Build history of the part. All positions in model axes, mm. Give positions to 0.01 mm unless a question says otherwise; leave off trailing zeros. Answer as a JSON object with one key per item and string values. Group by question number.
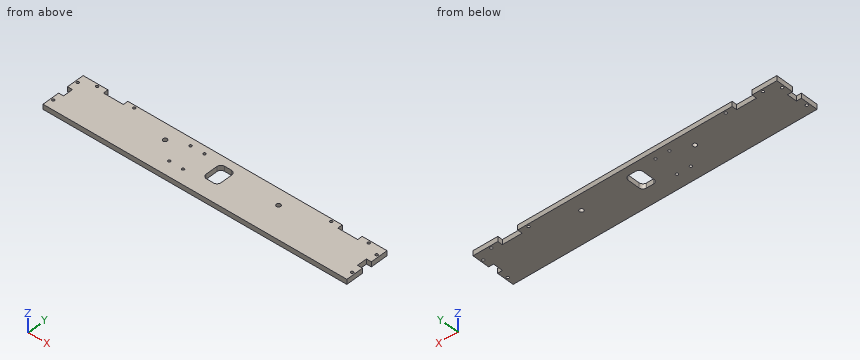
from build123d import *

# Parameters (mm, degrees)
SKETCH1_R           = 1.65
SKETCH1_R_2         = 2.7
BOSS_EXTRUDE1_DEPTH = 6.35
CUT_EXTRUDE1_REACH  = 8.35
SKETCH2_R           = 1.65


with BuildPart() as part:
    # Sketch1 → Boss-Extrude1 (new body)
    with BuildSketch(Plane(origin=(0, 0, 215.9), x_dir=(-1, 0, 0), z_dir=(0, 0, -1))):
        Polygon((50.8, 57.15), (50.8, 50.8), (25.4, 50.8), (25.4, 57.15), (-6.35, 57.15), (-6.35, 34.925), (0, 34.925), (0, 22.225), (-6.35, 22.225), (-6.35, 0), (382.27, 0), (382.27, 22.225), (375.92, 22.225), (375.92, 34.925), (382.27, 34.925), (382.27, 57.15), (350.52, 57.15), (350.52, 50.8), (325.12, 50.8), (325.12, 57.15), align=None)
        with Locations((379.095, 11.1125)):
            Circle(SKETCH1_R, mode=Mode.SUBTRACT)
        with Locations((-3.175, 11.1125)):
            Circle(SKETCH1_R, mode=Mode.SUBTRACT)
        with Locations((379.095, 46.037500912)):
            Circle(SKETCH1_R, mode=Mode.SUBTRACT)
        with Locations((-3.175, 46.037500912)):
            Circle(SKETCH1_R, mode=Mode.SUBTRACT)
        with Locations((314.0075, 53.975)):
            Circle(SKETCH1_R, mode=Mode.SUBTRACT)
        with Locations((61.9125, 53.975)):
            Circle(SKETCH1_R, mode=Mode.SUBTRACT)
        with Locations((361.6325, 53.975)):
            Circle(SKETCH1_R, mode=Mode.SUBTRACT)
        with Locations((14.2875, 53.975)):
            Circle(SKETCH1_R, mode=Mode.SUBTRACT)
        with Locations((260.51, 38.26)):
            Circle(SKETCH1_R_2, mode=Mode.SUBTRACT)
        with Locations((115.41, 38.26)):
            Circle(SKETCH1_R_2, mode=Mode.SUBTRACT)
        with BuildLine():
            Line((192.405, 21.59), (183.515, 21.59))
            ThreePointArc((183.515, 21.59), (179.922897552, 23.077897552), (178.435, 26.67))
            Line((178.435, 26.67), (178.435, 41.91))
            ThreePointArc((178.435, 41.91), (179.922897552, 45.502102448), (183.515, 46.99))
            Line((183.515, 46.99), (192.405, 46.99))
            ThreePointArc((192.405, 46.99), (195.997102448, 45.502102448), (197.485, 41.91))
            Line((197.485, 41.91), (197.485, 26.67))
            ThreePointArc((197.485, 26.67), (195.997102448, 23.077897552), (192.405, 21.59))
        make_face(mode=Mode.SUBTRACT)
    extrude(amount=-BOSS_EXTRUDE1_DEPTH)

    # Sketch2 → Cut-Extrude1 (cut, up to next)
    with BuildSketch(Plane.XY.offset(222.25), mode=Mode.PRIVATE) as cut_extrude1_sk1:
        with Locations((-218.821, 47.9552)):
            Circle(SKETCH2_R)
    cut_extrude1_tool1 = extrude(cut_extrude1_sk1.sketch, amount=-CUT_EXTRUDE1_REACH, mode=Mode.PRIVATE) & part.part
    add(cut_extrude1_tool1.solids().sort_by_distance((-218.821, 47.9552, 222.25))[0], mode=Mode.SUBTRACT)
    # Sketch2 → Cut-Extrude1 (cut, up to next)
    with BuildSketch(Plane.XY.offset(222.25), mode=Mode.PRIVATE) as cut_extrude1_sk2:
        with Locations((-236.601, 47.9552)):
            Circle(SKETCH2_R)
    cut_extrude1_tool2 = extrude(cut_extrude1_sk2.sketch, amount=-CUT_EXTRUDE1_REACH, mode=Mode.PRIVATE) & part.part
    add(cut_extrude1_tool2.solids().sort_by_distance((-236.601, 47.9552, 222.25))[0], mode=Mode.SUBTRACT)
    # Sketch2 → Cut-Extrude1 (cut, up to next)
    with BuildSketch(Plane.XY.offset(222.25), mode=Mode.PRIVATE) as cut_extrude1_sk3:
        with Locations((-236.601, 17.4752)):
            Circle(SKETCH2_R)
    cut_extrude1_tool3 = extrude(cut_extrude1_sk3.sketch, amount=-CUT_EXTRUDE1_REACH, mode=Mode.PRIVATE) & part.part
    add(cut_extrude1_tool3.solids().sort_by_distance((-236.601, 17.4752, 222.25))[0], mode=Mode.SUBTRACT)
    # Sketch2 → Cut-Extrude1 (cut, up to next)
    with BuildSketch(Plane.XY.offset(222.25), mode=Mode.PRIVATE) as cut_extrude1_sk4:
        with Locations((-218.821, 17.4752)):
            Circle(SKETCH2_R)
    cut_extrude1_tool4 = extrude(cut_extrude1_sk4.sketch, amount=-CUT_EXTRUDE1_REACH, mode=Mode.PRIVATE) & part.part
    add(cut_extrude1_tool4.solids().sort_by_distance((-218.821, 17.4752, 222.25))[0], mode=Mode.SUBTRACT)


solid = part.part
(1) Saw through at A-A on z = 220.5. Give the number of separate pieces and of enclosed holes in the cut face, plus the area to 3 significant figures.
(2) Pin check, flat tips, straight feed: pin 1 (2.5 mm diameter, centred on x = -236.6, y = 17.48, fed in from -Z); pin 2 (3 mm diameter, centred on x = -187.5, z = 218, fed in from -Y); pin 3 (2 mm diameter, centred on x = -336.5, z = 221, fed in from +Y); pin 4 (1.9 mm diameter, centred on y = 29, z = 218, fed in from -X). Stop position of each tip, or through.
(3) Probe line 1 along X through (y, z) = (38, 217) (3 decimals); line 2 along X through (y, z) = (52, 219.25); line 3 along X through (y, z) = (42, 216.5). List the from-to ranges inside material, lowest first. Write a range as [from, to].
Calculated:
{
 "1": {"separate pieces": "1", "enclosed holes": "15", "area": "21,100 mm^2"},
 "2": {"pin 1": "passes through", "pin 2": "stops at y = 0", "pin 3": "stops at y = 50.8", "pin 4": "stops at x = -375.92"},
 "3": {"line 1": "x = [-382.27, -263.197], [-257.823, -197.485], [-178.435, -118.097], [-112.723, 6.35]", "line 2": "x = [-382.27, -350.52], [-325.12, -50.8], [-25.4, 6.35]", "line 3": "x = [-382.27, -197.48], [-178.44, 6.35]"}
}
